For this review, take the finished solid that the model builds, in its own axes (mm). A direction names the side the tool comes from. Coordinates: 2 decimals unless noted, no trailing zeros. Write each loop counter-clockwise with the first axis right and the second up, starting at its lowest first coordinate (ties: lowest second). Pieces come first, ordered by that corner, then holes.
```python
from build123d import *

# Parameters (mm, degrees)
BOSS_EXTRUDE1_DEPTH = 15
SKETCH2_W           = 5
SKETCH2_H           = 4
CUT_EXTRUDE1_DEPTH  = 16
SKETCH7_R           = 1.75
CUT_EXTRUDE3_DEPTH  = 6


with BuildPart() as part:
    # Sketch1 → Boss-Extrude1 (new body)
    with BuildSketch(Plane.XY):
        Polygon((0, 36), (0, 0), (8.5, 0), (8.5, 20), (5, 20), (5, 36), align=None)
    extrude(amount=-BOSS_EXTRUDE1_DEPTH)

    # Sketch2 → Cut-Extrude1 (cut)
    with BuildSketch(Plane(origin=(0, 36, 0), x_dir=(1, 0, 0), z_dir=(0, 1, 0))):
        with Locations((2.5, 13)):
            Rectangle(SKETCH2_W, SKETCH2_H)
    extrude(amount=-CUT_EXTRUDE1_DEPTH, mode=Mode.SUBTRACT)

    # Sketch7 → Cut-Extrude3 (cut, through all)
    with BuildSketch(Plane(origin=(5, 0, 0), x_dir=(0, 0, -1), z_dir=(1, 0, 0))):
        with Locations((3, 33)):
            Circle(SKETCH7_R)
        with Locations((8, 33)):
            Circle(SKETCH7_R)
    extrude(amount=-CUT_EXTRUDE3_DEPTH, mode=Mode.SUBTRACT)


solid = part.part
```
Q1. Add section B-B (z = -8). State the section outline as (x, y) points, then the cut area to 4 significant figures.
Ans:
outline: (0, 0) - (8.5, 0) - (8.5, 20) - (5, 20) - (5, 31.25) - (0, 31.25) - close; (0, 34.75) - (5, 34.75) - (5, 36) - (0, 36) - close
area: 232.5 mm2
Q2. Add section A-A (y = 33). State the section outline as (x, z) points.
Ans:
outline: (0, -11) - (5, -11) - (5, -9.75) - (0, -9.75) - close; (0, -6.25) - (5, -6.25) - (5, -4.75) - (0, -4.75) - close; (0, -1.25) - (5, -1.25) - (5, 0) - (0, 0) - close
Q3. Add section D-D (z = -12.25). State the section outline as (x, y) points.
Ans:
outline: (0, 0) - (8.5, 0) - (8.5, 20) - (0, 20) - close
Q4. Tool access review of faces 1 (the flat face through (5, 28, -5)), 2 (the flat face through (8.5, 10, -7)): name each direction out of +Z, -Z, +X, -X, +Y, -Y from which nothing blocks a thin tool from reaching the whole face with its end or side.
Ans:
face 1: +Z, -Z, +X, +Y
face 2: +Z, -Z, +X, +Y, -Y
Q5. Draft analysis for pull direction Z (two halves, no side actions). For faces 3 (the cylindrical face through (2.5, 34.5, -8.9)), 4 (the flat face through (3, 14, 0)), 5 (the flat face through (0, 14, -7)), 6 (the flat face through (2, 28, -11)), state which applies: +Z half, -Z half, draft (parallel to the pull), parting line (faces both ways), or undercut.
Ans:
face 3: undercut
face 4: +Z half
face 5: draft
face 6: -Z half
Q6. Clearance check with a flat-ended pin moving along its axis: pin 1 Ø2 at (y, z) = (32, -1.5) entering from +X. State where the tip first meets the part, or that it passes through.
Ans:
pin 1: stops at x = 5
Q7. For probe 1 along Y at (x, z) = (1.1, -8); probe 2 along Y at (x, z) = (6.5, -0.75); probe 3 along Z at (x, y) = (3.25, 24), list the stretches that pass through material, from the lowest coordinate up.
Ans:
probe 1: y = 0 to 31.25, 34.75 to 36
probe 2: y = 0 to 20
probe 3: z = -11 to 0
Q8. Add section C-C (x = 3.5). State the section outline as (y, z) points.
Ans:
outline: (0, -15) - (20, -15) - (20, -11) - (36, -11) - (36, 0) - (0, 0) - close; hole circle Ø3.5 at (33, -8); hole circle Ø3.5 at (33, -3)
